Design review of the part shown in the three views and the two pictorial views. Dimensions are in mm from the part's minimum x, y and z. A direction names the side the tool comes from. Round coordinates to 2 decimals unless told otherwise and drop trailing zeros. Loops run counter-clockwise (first coordinate to the right, second up) from the corner with the lowest first, then second, coordinate; pieces in that order, holes last. Notation, with made-up numbers: M 64.25,19.25 L 113.25,19.25 A29 ccw 113.25,46.25 Z; hole C 89,49.5 d11. An arc over 180 degrees is marked long. Return JSON: item names as keys, results as strings. Group by question number.
Q1. For the marked faces 4, 5 and 6, list the 3-axis set-ups (+Z, -Z, +X, -X, +Y, -Y) from which the entire face can be reached by the end or side of a thin tool; tool diameter is ignored.
Q2. Clearance check with flat-ended pins moving along their axes: pin 1 Ø10 at (y, z) = (39, 15.5) entering from -X; pin 2 Ø5 at (y, z) = (15.5, 10) entering from -X; pin 3 Ø3 at (x, z) = (12.5, 9.5) entering from +Y; pin 4 Ø4 at (y, z) = (36.5, 15.5) entering from -X. State where each tip first meets the part, or that it passes through.
Q3. Consider section A-A (x = 38.1). State the section outline as (y, z) points.
Q4. Consider section C-C (y = 38.1). State the section outline as (x, z) points, and give its area (3 significant figures).
Q5. To check wall thickness, follow line 1 along Z through (x, y) = (4, 38.1); line 2 along X through (y, z) = (37.5, 13); line 3 along Y through (x, z) = (23, 13). State the ranges of each line that lie inside material, in increasing order.
Q6. Consider section B-B (z = 12.7). State the section outline as (x, y) points, and give its area (3 significant figures).
Q7. Consider section D-D (x = 7). State the section outline as (y, z) points.
Q8. Draft analysis for pull direction Z (two halves, no side actions). For the marked faces 1, 2 and 3, state which applies: pulls with the +Z half, pulls with the -Z half, needs draft (parallel to the pull), parting line crosses it, or undercut.
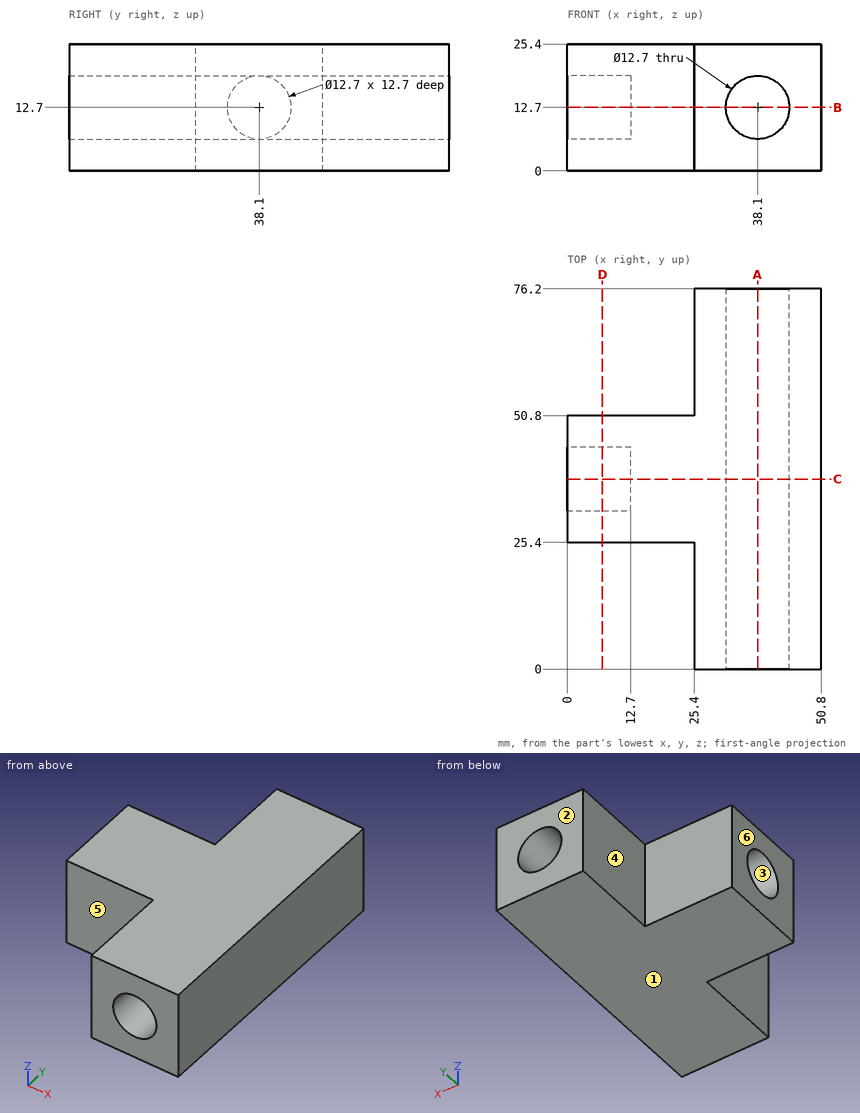
Values:
{
 "1": {"face 4": "+Z, -Z, -X, +Y", "face 5": "+Z, -Z, -X, -Y", "face 6": "+Z, -Z, -X, +Y, -Y"},
 "2": {"pin 1": "stops at x = 0", "pin 2": "stops at x = 25.4", "pin 3": "stops at y = 50.8", "pin 4": "stops at x = 12.7"},
 "3": {"outline": "M 0,0 L 76.2,0 L 76.2,6.35 L 0,6.35 Z; M 0,19.05 L 76.2,19.05 L 76.2,25.4 L 0,25.4 Z"},
 "4": {"outline": "M 0,0 L 50.8,0 L 50.8,25.4 L 0,25.4 L 0,19.05 L 12.7,19.05 L 12.7,6.35 L 0,6.35 Z; hole C 38.1,12.7 d12.7", "area": "1,000 mm2"},
 "5": {"line 1": "z = 0 to 6.35, 19.05 to 25.4", "line 2": "x = 12.7 to 31.76, 44.44 to 50.8", "line 3": "y = 25.4 to 50.8"},
 "6": {"outline": "M 0,25.4 L 25.4,25.4 L 25.4,0 L 31.75,0 L 31.75,76.2 L 25.4,76.2 L 25.4,50.8 L 0,50.8 L 0,44.45 L 12.7,44.45 L 12.7,31.75 L 0,31.75 Z; M 44.45,0 L 50.8,0 L 50.8,76.2 L 44.45,76.2 Z", "area": "1,450 mm2"},
 "7": {"outline": "M 25.4,0 L 50.8,0 L 50.8,25.4 L 25.4,25.4 Z; hole C 38.1,12.7 d12.7"},
 "8": {"face 1": "pulls with the -Z half", "face 2": "needs draft", "face 3": "undercut"}
}
